Geometry check sheet. Reference: the model listing, model coordinates, mm. Coordinates: 2 decimals unless noted, no trailing zeros. Loops run counter-clockwise (first coordinate to the right, second up) from the corner with the lowest first, then second, coordinate; pieces in that order, holes last.
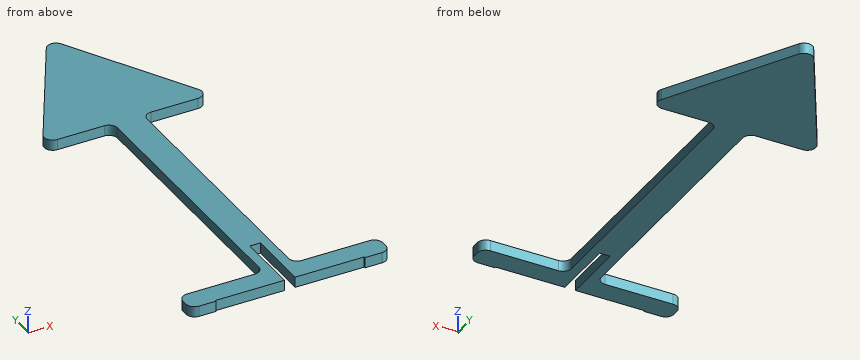
from build123d import *

# Parameters (mm, degrees)
F0_W     = 6
F0_H     = 0.3
F1_DEPTH = 2.5
F2_R     = 2


with BuildPart() as f1:
    # F0 (on Top) → F1 (new body)
    with BuildSketch(Plane.XY):
        Polygon((0, 35), (-20, 0), (-3.5, 0), (3.5, 0), (20, 0), align=None)
        Polygon((3.5, 0), (-3.5, 0), (-3.5, -65), (-23.5, -65), (-23.5, -70), (-17.5, -70), (-1.25, -70), (-1.25, -55), (1.25, -55), (1.25, -70), (17.5, -70), (23.5, -70), (23.5, -65), (3.5, -65), align=None)
        with Locations((-20.5, -70.15)):
            Rectangle(F0_W, F0_H)
        with Locations((20.5, -70.15)):
            Rectangle(F0_W, F0_H)
    extrude(amount=F1_DEPTH)

    # F2
    f2_edges = [f1.edges().sort_by_distance(p)[0] for p in [
        (-3.5, 0, 1.25),
        (3.5, 0, 1.25),
        (20, 0, 1.25),
        (-20, 0, 1.25),
        (0, 35, 1.25),
        (3.5, -65, 1.25),
        (-3.5, -65, 1.25),
        (-23.5, -65, 1.25),
        (23.5, -65, 1.25),
        (-23.5, -70.3, 1.25),
        (23.5, -70.3, 1.25),
    ]]
    fillet(f2_edges, radius=F2_R)


solid = f1.part
(1) Gauge pin test, flat ends, axial feed: pin 1 Ø1.5 at (x, z) = (-6, 1) entering from +Y; pin 2 Ø5 at (x, y) = (14.5, -1) entering from -Z; pin 3 Ø1.2 at (y, z) = (-39.5, 1) entering from -X; pin 4 Ø1 at (x, z) = (9.5, 0.5) entering from +Y. Record the tip position at first contact, or that the pin passes through.
Findings:
pin 1: stops at y = 25.81
pin 2: stops at z = 0
pin 3: stops at x = -3.5
pin 4: stops at y = 19.25
(2) Scan lines: L1, parallel to X at y = -62, z = 0.4; L2, parallel to X at y = 3, z = 0.9; L3, parallel to X at y = -39.5, z = 0.8. Record each from-to range of solid material in increasing order.
Findings:
L1: x = -3.5 to -1.25, 1.25 to 3.5
L2: x = -18.29 to 18.29
L3: x = -3.5 to 3.5
(3) Sectioned sample at B-B on y = -58. Record the cut outline in (x, z).
Findings:
outline: (-3.5, 0) - (-1.25, 0) - (-1.25, 2.5) - (-3.5, 2.5) - close; (1.25, 0) - (3.5, 0) - (3.5, 2.5) - (1.25, 2.5) - close
(4) Sectioned sample at D-D on x = -20. Record the cut outline in (y, z), and give its area (4 significant figures).
Findings:
outline: (-70.3, 0) - (-65, 0) - (-65, 2.5) - (-70.3, 2.5) - close
area: 13.25 mm2
(5) Sectioned sample at A-A on x = 15. Record the cut outline in (y, z).
Findings:
outline: (-70, 0) - (-65, 0) - (-65, 2.5) - (-70, 2.5) - close; (0, 0) - (8.75, 0) - (8.75, 2.5) - (0, 2.5) - close
